Autodesk Fusion 360 part; units mm, degrees
sketch "Sketch2" plane through (0, 0, 0) normal (0, 1, 0) x (1, 0, 0)
  circle A0 centre (-68.199, 28.575) radius 5.588
  circle A1 centre (-68.199, -28.575) radius 5.588
  circle A2 centre (68.199, -28.575) radius 5.588
  circle A3 centre (68.199, 28.575) radius 5.588
  circle A4 centre (68.199, 28.575) radius 12.7
  circle A5 centre (68.199, -28.575) radius 12.7
  circle A6 centre (-68.199, 28.575) radius 12.7
  circle A7 centre (-68.199, -28.575) radius 12.7
  line L0 (-80.899, 28.575) -> (-80.899, -28.575)
  line L1 (68.199, -41.275) -> (-68.199, -41.275)
  line L2 (80.899, 28.575) -> (80.899, -28.575)
  line L3 (68.199, 41.275) -> (-68.199, 41.275)
  line L4 (68.199, -28.575) -> (56.4856, -23.6672) construction
  line L5 (-36.449, 41.275) -> (-36.449, -41.275)
  line L6 (36.449, -41.275) -> (36.449, 41.275)
  line L7 (56.4856, 23.6672) -> (68.199, 28.575) construction
  dimension "d19" = 136.398
  dimension "d20" = 57.15
  dimension "d21" = 11.176
  dimension "d22" = 11.176
  dimension "d23" = 11.176
  dimension "d24" = 11.176
  dimension "d25" = 25.4
  dimension "d26" = 25.4
  dimension "d27" = 25.4
  dimension "d28" = 25.4
extrude "Extrude5" add sketch "Sketch2" along normal blind 15.748 contours L1 L3 L5 L6 makes body 1
extrude "Extrude4" add sketch "Sketch2" along normal blind 12.7 separate body contours A4 | A4 A5 L1 L2 L3 L6 | A5 | A6 A7 L0 L1 L3 L5 | A6 | A7 makes body 2 at (-45.4933, 0, 8.4757) makes body 3 at (45.4933, 0, 8.4757)
extrude "Extrude6" cut sketch "Sketch2" along normal blind 3.302 contours L1 L3 L5 L6 bodies 1
combine "Combine2" operation add target body 3 tool bodies 1 2
Read the model definition and answer for the solid it produces. Units are mm, in the model's axes. A direction names the side the tool comes from. Coordinates: 2 decimals unless noted, no trailing zeros. Write each loop counter-clockwise with the first axis right and the second up, starting at its lowest first coordinate (ties: lowest second). Pieces come first, ordered by that corner, then holes. Notation, with made-up numbers: (50, -15.5) - (85, -15.5) arc R12 ccw to (85, 5.5) - close; hole circle Ø9 at (34, 3.5). An arc over 180 degrees is marked (long way). One line per question, with ' | ' between items.
Q1. Find section A-A, the plane y = 1.5. Write down the section's boundary in (x, z) (3 decimals).
Result set:
outline: (-80.899, -28.575) arc R12.7 ccw to (-68.199, -41.275) - (-36.449, -41.275) - (-36.449, 41.275) - (-68.199, 41.275) arc R12.7 ccw to (-80.899, 28.575) - close; (36.449, -41.275) - (68.199, -41.275) arc R12.7 ccw to (80.899, -28.575) - (80.899, 28.575) arc R12.7 ccw to (68.199, 41.275) - (36.449, 41.275) - close; hole circle Ø11.176 at (-68.199, -28.575); hole circle Ø11.176 at (-68.199, 28.575); hole circle Ø11.176 at (68.199, -28.575); hole circle Ø11.176 at (68.199, 28.575)
Q2. Consider L1, parallel to Z at x = 72, y = 6; L2, parallel to Y at x = -51, z = -32; L3, parallel to X at y = 13, z = -12. Determine where each line is inside the solid, lowest interval first. Write a range as [from, to].
Result set:
L1: [-40.69, -32.67], [-24.48, 24.48], [32.67, 40.69] | L2: [0, 12.7] | L3: [-36.45, 36.45]
Q3. Determine the mould class of faces 1 (the flat face through (58, 12.7, -1)), 2 (the flat face through (-1, 3.302, -1)), 3 (the cylindrical face through (77.08, 6.261, -37.653)) for opening direction X: +X half, -X half, draft (parallel to the pull), parting line (faces both ways), or undercut.
Result set:
face 1: draft | face 2: undercut | face 3: +X half
Q4. Find section D-D, the plane z = -12. Write down the section's boundary in (x, y), plus the area to 3 significant figures.
Result set:
outline: (-80.9, 0) - (-36.45, 0) - (-36.45, 3.3) - (36.45, 3.3) - (36.45, 0) - (80.9, 0) - (80.9, 12.7) - (36.45, 12.7) - (36.45, 15.75) - (-36.45, 15.75) - (-36.45, 12.7) - (-80.9, 12.7) - close | area: 2,040 mm^2
Q5. Each of these flat-tipped pins is pushed along its axis until it touches: P1, Ø1.5, axis at y = 15, z = 6.5, coming from the -X side; P2, Ø1, axis at x = 29, z = 3, coming from the -Y side; P3, Ø0.9, axis at y = 15, z = -15.5, coming from the +X side; P4, Ø1.5, axis at x = 48, z = -21.5, coming from the -Y side. Where does it stop, or does it pass through?
Result set:
P1: x = -36.45 | P2: y = 3.3 | P3: x = 36.45 | P4: y = 0
Q6. Find section B-B, the plane z = -25. Write down the section's boundary in (x, y).
Result set:
outline: (-80.9, 0) - (-72.49, 0) - (-72.49, 12.7) - (-80.9, 12.7) - close; (-63.9, 0) - (-36.45, 0) - (-36.45, 3.3) - (36.45, 3.3) - (36.45, 0) - (63.9, 0) - (63.9, 12.7) - (36.45, 12.7) - (36.45, 15.75) - (-36.45, 15.75) - (-36.45, 12.7) - (-63.9, 12.7) - close; (72.49, 0) - (80.9, 0) - (80.9, 12.7) - (72.49, 12.7) - close
Q7. Find section C-C, the plane x = -66.5. Write down the section's boundary in (y, z) (3 decimals), plus the area to 3 significant figures.
Result set:
outline: (0, -41.275) - (12.7, -41.275) - (12.7, -33.898) - (0, -33.898) - close; (0, -23.252) - (12.7, -23.252) - (12.7, 23.252) - (0, 23.252) - close; (0, 33.898) - (12.7, 33.898) - (12.7, 41.275) - (0, 41.275) - close | area: 778 mm^2
Q8. For faces 4 (the flat face through (36.449, 14, 1)), 5 (the cylindrical face through (-77.277, 6.261, -37.456)), 6 (the flat face through (36.449, 2, 1)), 7 (the flat face through (-36.449, 14, -1)), determine the directions among +Z, -Z, +X, -X, +Y, -Y from which every point of the face is accessible in a straight line to the end or side of a thin tool.
Result set:
face 4: +Z, -Z, +X, +Y | face 5: -Z, -X, +Y, -Y | face 6: +Z, -Z, -Y | face 7: +Z, -Z, -X, +Y
